Design review of the part built by this model. Coordinates are the model's own, in mm. Face numbers are marked on the shaded views. A direction names the side the tool comes from. Give positions to 0.01 mm unless a question says otherwise; leave off trailing zeros. Order: outer loops, then holes, each group sorted by start corner. A loop starts at its lowest first (then second) coordinate and runs counter-clockwise, first axis right, second up.
```python
from build123d import *

# Parameters (mm, degrees)
SKETCH1_R            = 15
BOSS_EXTRUDE2_DEPTH  = 8.255
BOSS_EXTRUDE3_DEPTH  = 8.255
BOSS_EXTRUDE4_DEPTH  = 38.1
SKETCH5_R            = 3.249999977
CUT_EXTRUDE3_DEPTH   = 63.5
BOSS_EXTRUDE13_DEPTH = 3.175
BOSS_EXTRUDE14_DEPTH = 3.175
BOSS_EXTRUDE15_DEPTH = 3.175
CUT_EXTRUDE6_DEPTH   = 9.255
SKETCH20_W           = 38.1
SKETCH20_H           = 44.45
BOSS_EXTRUDE16_DEPTH = 1.524
SKETCH21_W           = 38.1
SKETCH21_H           = 44.45
BOSS_EXTRUDE17_DEPTH = 1.524
SKETCH23_R           = 1.9431
CUT_EXTRUDE7_DEPTH   = 2.54
SKETCH24_R           = 1.98501
CUT_EXTRUDE8_DEPTH   = 2.54
SKETCH25_W           = 19.05
SKETCH25_H           = 38.1
BOSS_EXTRUDE18_DEPTH = 1.587961
SKETCH26_W           = 19.05
SKETCH26_H           = 38.1
BOSS_EXTRUDE19_DEPTH = 1.587961
BOSS_EXTRUDE20_START = -0.60614
SKETCH27_W           = 25.4
SKETCH27_H           = 22.811309973
BOSS_EXTRUDE20_DEPTH = 0.60614
CUT_EXTRUDE9_REACH   = 202.702
SKETCH29_R           = 1.524
CUT_EXTRUDE10_REACH  = 202.702
SKETCH30_W           = 6.954293398
SKETCH30_H           = 5.349239075


with BuildPart() as part:
    # Sketch1 → Boss-Extrude2 (new body)
    with BuildSketch(Plane(origin=(0, 0, 0), x_dir=(1, 0, 0), z_dir=(0, 1, 0))):
        Circle(SKETCH1_R)
    extrude(amount=BOSS_EXTRUDE2_DEPTH)

    # Sketch1<6> → Boss-Extrude3 (add)
    with BuildSketch(Plane(origin=(0, 0, 0), x_dir=(1, 0, 0), z_dir=(0, 1, 0))):
        with BuildLine():
            ThreePointArc((3.175, 130.136274728), (1.587618078, 130.165318322), (0, 130.175))
            Line((0, 130.175), (0, 15))
            ThreePointArc((0, 15), (1.596569562, 14.914790164), (3.175, 14.660128751))
            Line((3.175, 14.660128751), (3.175, 130.136274728))
        make_face()
        with BuildLine():
            Line((-9.42450178, 11.66956581), (-90.918248264, 93.163312294))
            ThreePointArc((-90.918248264, 93.163312294), (-92.047625241, 92.047625241), (-93.163312294, 90.918248264))
            Line((-93.163312294, 90.918248264), (-11.66956581, 9.42450178))
            ThreePointArc((-11.66956581, 9.42450178), (-10.606601718, 10.606601718), (-9.42450178, 11.66956581))
        make_face()
        with BuildLine():
            Line((-15, 0), (-130.175, 0))
            ThreePointArc((-130.175, 0), (-130.165318322, -1.587618078), (-130.136274728, -3.175))
            Line((-130.136274728, -3.175), (-14.660128751, -3.175))
            ThreePointArc((-14.660128751, -3.175), (-14.914790164, -1.596569562), (-15, 0))
        make_face()
    extrude(amount=BOSS_EXTRUDE3_DEPTH)

    # Sketch1<7> → Boss-Extrude4 (add)
    with BuildSketch(Plane(origin=(0, 0, 0), x_dir=(1, 0, 0), z_dir=(0, 1, 0))):
        with BuildLine():
            Line((3.175, 130.136274728), (3.175, 133.312197023))
            ThreePointArc((3.175, 133.312197023), (-94.292689271, 94.292689271), (-133.312197023, -3.175))
            Line((-133.312197023, -3.175), (-130.136274728, -3.175))
            ThreePointArc((-130.136274728, -3.175), (-92.047625241, 92.047625241), (3.175, 130.136274728))
        make_face()
    extrude(amount=BOSS_EXTRUDE4_DEPTH)

    # Sketch5 → Cut-Extrude3 (cut)
    with BuildSketch(Plane(origin=(0, 8.255, 0), x_dir=(1, 0, 0), z_dir=(0, 1, 0))):
        Circle(SKETCH5_R)
    extrude(amount=-CUT_EXTRUDE3_DEPTH, mode=Mode.SUBTRACT)

    # Sketch14 → Boss-Extrude13 (add)
    with BuildSketch(Plane(origin=(0, 0, 0), x_dir=(-1, 0, 0), z_dir=(0, 0, -1))):
        Polygon((130.175, 8.255), (111.125, 8.255), (130.175, 27.305), align=None)
    extrude(amount=-BOSS_EXTRUDE13_DEPTH)

    # Sketch15 → Boss-Extrude14 (add)
    with BuildSketch(Plane.ZY):
        Polygon((-130.175, 8.255), (-130.175, 27.305), (-111.125, 8.255), align=None)
    extrude(amount=-BOSS_EXTRUDE14_DEPTH)

    # Sketch16 → Boss-Extrude15 (add)
    with BuildSketch(Plane(origin=(1.122532015, 0, -1.122532015), x_dir=(-0.707106781, 0, -0.707106781), z_dir=(0.707106781, 0, -0.707106781))):
        Polygon((133.340319762, 8.255), (111.115319762, 8.255), (133.340319762, 27.305), align=None)
    extrude(amount=-BOSS_EXTRUDE15_DEPTH)

    # Sketch17 → Cut-Extrude6 (cut, through all)
    with BuildSketch(Plane(origin=(0, 8.255, 0), x_dir=(1, 0, 0), z_dir=(0, 1, 0))):
        with BuildLine():
            Line((-5.908712478, 5.423058993), (-7.721732332, 7.873214705))
            ThreePointArc((-7.721732332, 7.873214705), (-7.403164404, 10.004802487), (-5.271576621, 9.686234559))
            Line((-5.271576621, 9.686234559), (-3.458556767, 7.236078848))
            ThreePointArc((-3.458556767, 7.236078848), (-3.777124696, 5.104491065), (-5.908712478, 5.423058993))
        make_face()
        with BuildLine():
            Line((3.458556767, -7.236078848), (5.271576621, -9.686234559))
            ThreePointArc((5.271576621, -9.686234559), (7.403164404, -10.004802487), (7.721732332, -7.873214705))
            Line((7.721732332, -7.873214705), (5.908712478, -5.423058993))
            ThreePointArc((5.908712478, -5.423058993), (3.777124696, -5.104491065), (3.458556767, -7.236078848))
        make_face()
    extrude(amount=-CUT_EXTRUDE6_DEPTH, mode=Mode.SUBTRACT)

    # Sketch20 → Boss-Extrude16 (add)
    with BuildSketch(Plane(origin=(0, 0, -131.724235875), x_dir=(0, -1, 0), z_dir=(0, 0, -1))):
        with Locations((-19.05, -25.4)):
            Rectangle(SKETCH20_W, SKETCH20_H)
    extrude(amount=-BOSS_EXTRUDE16_DEPTH)

    # Sketch21 → Boss-Extrude17 (add)
    with BuildSketch(Plane(origin=(-131.724235875, 0, 0), x_dir=(0, -1, 0), z_dir=(-1, 0, 0))):
        with Locations((-19.05, 25.4)):
            Rectangle(SKETCH21_W, SKETCH21_H)
    extrude(amount=-BOSS_EXTRUDE17_DEPTH)

    # Sketch23 → Cut-Extrude7 (cut)
    with BuildSketch(Plane.ZY.offset(131.724235875)):
        with Locations((34.925, 31.75)):
            Circle(SKETCH23_R)
        with Locations((34.925, 6.35)):
            Circle(SKETCH23_R)
    extrude(amount=-CUT_EXTRUDE7_DEPTH, mode=Mode.SUBTRACT)

    # Sketch24 → Cut-Extrude8 (cut)
    with BuildSketch(Plane(origin=(0, 0, -131.724235875), x_dir=(-1, 0, 0), z_dir=(0, 0, -1))):
        with Locations((-34.925, 31.75)):
            Circle(SKETCH24_R)
        with Locations((-34.925, 6.35)):
            Circle(SKETCH24_R)
    extrude(amount=-CUT_EXTRUDE8_DEPTH, mode=Mode.SUBTRACT)

    # Sketch25 → Boss-Extrude18 (add)
    with BuildSketch(Plane.ZY.offset(131.724235875)):
        with Locations((12.7, 19.05)):
            Rectangle(SKETCH25_W, SKETCH25_H)
    extrude(amount=BOSS_EXTRUDE18_DEPTH)

    # Sketch26 → Boss-Extrude19 (add)
    with BuildSketch(Plane(origin=(0, 0, -131.724235875), x_dir=(-1, 0, 0), z_dir=(0, 0, -1))):
        with Locations((-12.7, 19.05)):
            Rectangle(SKETCH26_W, SKETCH26_H)
    extrude(amount=BOSS_EXTRUDE19_DEPTH)

    # Sketch27 → Boss-Extrude20 (add)
    with BuildSketch(Plane(origin=(-94.292689271, 0, -94.292689271), x_dir=(-0.707106781, 0, 0.707106781), z_dir=(-0.707106781, 0, -0.707106781)).offset(BOSS_EXTRUDE20_START)):
        with Locations((0, 11.405654987)):
            Rectangle(SKETCH27_W, SKETCH27_H)
    extrude(amount=BOSS_EXTRUDE20_DEPTH)

    # Sketch29 → Cut-Extrude9 (cut, up to next)
    with BuildSketch(Plane(origin=(-94.292689271, 0, -94.292689271), x_dir=(-0.707106781, 0, 0.707106781), z_dir=(-0.707106781, 0, -0.707106781)), mode=Mode.PRIVATE) as cut_extrude9_sk1:
        with Locations((8.636, 4.064)):
            Circle(SKETCH29_R)
    cut_extrude9_tool1 = extrude(cut_extrude9_sk1.sketch, amount=-CUT_EXTRUDE9_REACH, mode=Mode.PRIVATE) & part.part
    add(cut_extrude9_tool1.solids().sort_by_distance((-100.399263, 4.064, -88.186115))[0], mode=Mode.SUBTRACT)
    # Sketch29 → Cut-Extrude9 (cut, up to next)
    with BuildSketch(Plane(origin=(-94.292689271, 0, -94.292689271), x_dir=(-0.707106781, 0, 0.707106781), z_dir=(-0.707106781, 0, -0.707106781)), mode=Mode.PRIVATE) as cut_extrude9_sk2:
        with Locations((-8.636, 18.747309973)):
            Circle(SKETCH29_R)
    cut_extrude9_tool2 = extrude(cut_extrude9_sk2.sketch, amount=-CUT_EXTRUDE9_REACH, mode=Mode.PRIVATE) & part.part
    add(cut_extrude9_tool2.solids().sort_by_distance((-88.186115, 18.74731, -100.399263))[0], mode=Mode.SUBTRACT)

    # Sketch30 → Cut-Extrude10 (cut, up to next)
    with BuildSketch(Plane(origin=(-94.292689271, 0, -94.292689271), x_dir=(-0.707106781, 0, 0.707106781), z_dir=(-0.707106781, 0, -0.707106781)), mode=Mode.PRIVATE) as cut_extrude10_sk1:
        with Locations((6.047853301, 13.786690436)):
            Rectangle(SKETCH30_W, SKETCH30_H)
    cut_extrude10_tool1 = extrude(cut_extrude10_sk1.sketch, amount=-CUT_EXTRUDE10_REACH, mode=Mode.PRIVATE) & part.part
    add(cut_extrude10_tool1.solids().sort_by_distance((-98.569167, 13.78669, -90.016211))[0], mode=Mode.SUBTRACT)


solid = part.part
```
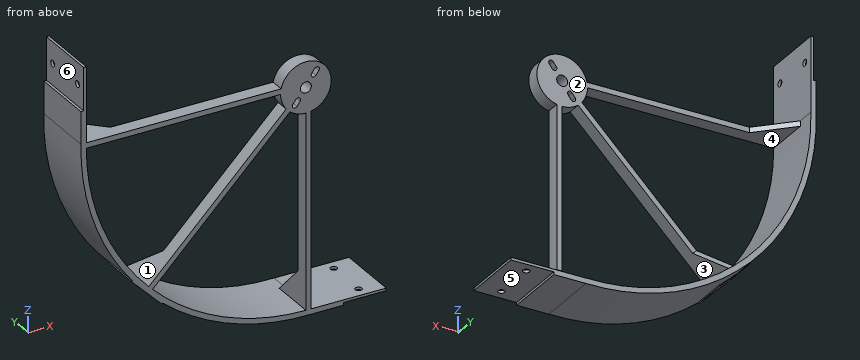
1. Machinability: for the marked faces 1 and 2, which of the approach directions +Z, -Z, +X, -X, +Y, -Y give a long, thin tool a straight path to every point of the face, cutting with its end or side? Answer none if there is none.
Recorded:
face 1: +Y, -Y
face 2: +Z, +X, +Y
2. Take a section at C-C (x = -72.5). State the section outline as (y, z) points (1 decimal).
Recorded:
outline: (0, -111.9) - (38.1, -111.9) - (38.1, -108.1) - (0, -108.1) - close; (0, -74.7) - (8.3, -74.7) - (8.3, -70.3) - (0, -70.3) - close; (0, 0) - (8.3, 0) - (8.3, 3.2) - (0, 3.2) - close
3. Take a section at D-D (x = -106). State the section outline as (y, z) points (3 decimals).
Recorded:
outline: (0, -80.909) - (38.1, -80.909) - (38.1, -75.561) - (0, -75.561) - close; (0, 0) - (8.255, 0) - (8.255, 3.175) - (0, 3.175) - close
4. Take a section at B-B (z = -69). State the section outline as (x, y) points (3 decimals).
Recorded:
outline: (-114.111, 0) - (-110.384, 0) - (-110.384, 38.1) - (-114.111, 38.1) - close; (-71.245, 0) - (-66.755, 0) - (-66.755, 8.255) - (-71.245, 8.255) - close; (0, 0) - (3.175, 0) - (3.175, 8.255) - (0, 8.255) - close
5. Take a section at A-A (x = 12). State the section outline as (y, z) points (3 decimals).
Recorded:
outline: (0, -133.312) - (38.1, -133.312) - (38.1, -130.2) - (0, -130.2) - close; (0, -9) - (8.255, -9) - (8.255, 9) - (0, 9) - close
6. For line 1 along X through (y, z) = (8, -69) (3 decimals); line 2 along X through (y, z) = (5, -61) (3 decimals); line 3 along Z through (x, y) = (-46.5, 5.5) (3 decimals), list the stretches that pass through material, from the lowest coordinate up.
Recorded:
line 1: x = -114.111 to -110.384, -71.245 to -66.755, 0 to 3.175
line 2: x = -118.58 to -114.998, -63.245 to -58.755, 0 to 3.175
line 3: z = -124.98 to -121.587, -48.745 to -44.255, 0 to 3.175
7. Draft analysis for pull direction X (two halves, no side actions). For the marked faces 3, 4, 5 and 6, state which applies: pulls with the +X half, pulls with the -X half, needs draft (parallel to the pull), parting line crosses it, or undercut.
Recorded:
face 3: undercut
face 4: undercut
face 5: needs draft
face 6: pulls with the -X half
8. For pin 1 (4 mm diameter, centred on y = 21.5, z = -7.5, fed in from -X); pin 2 (3 mm diameter, centred on x = 34.925, y = 6.35, fed in from +Z) (1 decimal); pin 3 (3 mm diameter, centred on x = -47, y = 10, fed in from +Z); pin 4 (5.5 mm diameter, centred on y = 10, z = 9, fed in from -X), all flat-tipped, find the tip position at first contact; note any pin that passes through.
Recorded:
pin 1: stops at x = -133.24
pin 2: passes through
pin 3: stops at z = -120.8
pin 4: stops at x = -133.31
